The model under review builds one solid part; all positions refer to its coordinate system, in mm. A direction names the side the tool comes from. Coordinates: 2 decimals unless noted, no trailing zeros. Order: outer loops, then holes, each group sorted by start corner. A loop starts at its lowest first (then second) coordinate and runs counter-clockwise, first axis right, second up. Notation, with made-up numbers: (83.5, 88) - (100.5, 88) arc R16 ccw to (100.5, 95) - close; hole circle Ø5 at (67, 58.5). An arc over 180 degrees is marked (long way). Answer in a Markdown table with one row per item.
```python
from build123d import *

# Parameters (mm, degrees)
F1_DEPTH  = 32
F3_DEPTH  = 13.001
F4_R      = 5.5
F5_DEPTH  = 13.001
F6_R      = 6.5
F7_DEPTH  = 88.001
F9_DEPTH  = 88.001
F10_DEPTH = 88.001


with BuildPart() as f1:
    # F0 (on Front) → F1 (new body)
    with BuildSketch(Plane.XZ):
        Polygon((-39, 0), (0, 0), (0, 13), (35, 13), (35, 0), (74, 0), (74, 13), (49, 13), (49, 64), (30, 64), (30, 26), (5, 26), (5, 64), (-14, 64), (-14, 13), (-39, 13), align=None)
    extrude(amount=F1_DEPTH)

    # F2 (on face) → F3 (cut, through all)
    with BuildSketch(Plane.XY.offset(13)):
        Polygon((74, -22), (64, -32), (74, -32), align=None)
        Polygon((-39, -32), (-29, -32), (-39, -22), align=None)
    extrude(amount=-F3_DEPTH, mode=Mode.SUBTRACT)

    # F4 (on face) → F5 (cut, through all)
    with BuildSketch(Plane.XY.offset(13)):
        with Locations((-26, -13)):
            Circle(F4_R)
        with Locations((61, -13)):
            Circle(F4_R)
    extrude(amount=-F5_DEPTH, mode=Mode.SUBTRACT)

    # F6 (on face) → F7 (cut, through all)
    with BuildSketch(Plane.YZ.offset(49)):
        with Locations((-16, 46)):
            Circle(F6_R)
    extrude(amount=-F7_DEPTH, mode=Mode.SUBTRACT)

    # F8 (on face) → F9 (cut, through all)
    with BuildSketch(Plane.YZ.offset(49)):
        with BuildLine():
            ThreePointArc((-32, 60.128765), (-24.230833, 63.018427), (-16, 64))
            Line((-16, 64), (-32, 64))
            Line((-32, 64), (-32, 60.128765))
        make_face()
        with BuildLine():
            ThreePointArc((-16, 64), (-7.769167, 63.018427), (0, 60.128765))
            Line((0, 60.128765), (0, 64))
            Line((0, 64), (-16, 64))
        make_face()
    extrude(amount=-F9_DEPTH, mode=Mode.SUBTRACT)

    # F8 (on face) → F10 (cut, through all)
    with BuildSketch(Plane.YZ.offset(49)):
        with BuildLine():
            ThreePointArc((-32, 60.128765), (-24.230833, 63.018427), (-16, 64))
            Line((-16, 64), (-32, 64))
            Line((-32, 64), (-32, 60.128765))
        make_face()
        with BuildLine():
            ThreePointArc((-16, 64), (-7.769167, 63.018427), (0, 60.128765))
            Line((0, 60.128765), (0, 64))
            Line((0, 64), (-16, 64))
        make_face()
    extrude(amount=-F10_DEPTH, mode=Mode.SUBTRACT)


solid = f1.part
```
Item 1: We need section C-C, the plane y = -13. State how many separate pieces and enclosed holes the cut face has, then the cut area to 3 significant figures.
Check values:
| item | result |
|---|---|
| separate pieces | 5 |
| enclosed holes | 0 |
| area | 2,550 mm^2 |
Item 2: We need section B-B, the plane x = -26. Write out the cut boundary in (y, z), then the cut area to 3 significant figures.
Check values:
| item | result |
|---|---|
| outline | (-32, 0) - (-18.5, 0) - (-18.5, 13) - (-32, 13) - close; (-7.5, 0) - (0, 0) - (0, 13) - (-7.5, 13) - close |
| area | 273 mm^2 |
Item 3: We need section D-D, the plane x = 33.5. Write out the cut boundary in (y, z).
Check values:
| item | result |
|---|---|
| outline | (-32, 13) - (0, 13) - (0, 60.13) arc R35 ccw to (-16, 64) arc R35 ccw to (-32, 60.13) - close; hole circle Ø13 at (-16, 46) |
Item 4: Mouldability with a two-part tool opening along Y and no side actions: class faces 4 (the face through (5, -12.2, 40.5)), 5 (the face through (27, -32, 24)), 6 (the face through (17, 0, 24)), 7 (the face through (39.633, -22.494, 46.286)) as +Y half, -Y half, draft (parallel to the pull), parting line (faces both ways), or undercut.
Check values:
| item | result |
|---|---|
| face 4 | draft |
| face 5 | -Y half |
| face 6 | +Y half |
| face 7 | undercut |
Item 5: Tool access review of faces 1 (the face through (-14, -16, 39)), 2 (the face through (62, -19, 13)), 3 (the face through (30, -23, 45)): name each direction out of +Z, -Z, +X, -X, +Y, -Y from which nothing blocks a thin tool from reaching the whole face with its end or side.
Check values:
| item | result |
|---|---|
| face 1 | +Z, -X, +Y, -Y |
| face 2 | +Z, +X, +Y, -Y |
| face 3 | +Z, +Y, -Y |
Item 6: Clearance check with flat-ended pins moving along their axes: pin 1 Ø16 at (y, z) = (-22, 31.5) entering from -X; pin 2 Ø12.5 at (x, y) = (-32, -14.5) entering from +Z; pin 3 Ø12 at (y, z) = (-8, 30.5) entering from +X. State where each tip first meets the part, or that it passes through.
Check values:
| item | result |
|---|---|
| pin 1 | x = -14 |
| pin 2 | z = 13 |
| pin 3 | x = 49 |
Item 7: We need section A-A, the plane z = 9. Write out the cut boundary in (x, y), then the cut area to 3 significant figures.
Check values:
| item | result |
|---|---|
| outline | (-39, -22) - (-29, -32) - (0, -32) - (0, 0) - (-39, 0) - close; (35, -32) - (64, -32) - (74, -22) - (74, 0) - (35, 0) - close; hole circle Ø11 at (-26, -13); hole circle Ø11 at (61, -13) |
| area | 2,210 mm^2 |
Item 8: To check wall thickness, follow line 1 (X direction, y = -25, z = 55); line 2 (Y direction, x = 61, z = 5.75); line 3 (X direction, y = -10.5, z = 9). State the ranges of each line that lie inside material, in increasing order. Write a range as from..to.
Check values:
| item | result |
|---|---|
| line 1 | -14..5, 30..49 |
| line 2 | -32..-18.5, -7.5..0 |
| line 3 | -39..-30.9, -21.1..0, 35..56.1, 65.9..74 |
